Here's the drawing with two shaded views (mm, measured from the low corner). I have some questions. A direction names the side the tool comes from. Coordinates: 2 decimals unless noted, no trailing zeros. Order: outer loops, then holes, each group sorted by start corner. A loop starts at its lowest first (then second) coordinate and runs counter-clockwise, first axis right, second up. Notation, with made-up numbers: (9.25, 84) - (56.25, 84) arc R29 cw to (56.25, 117) - close; hole circle Ø4 at (13, 47.5). An arc over 180 degrees is marked (long way). Answer as CSV lines item,"result". Start each with the question number.
1. I want a section at D-D, the plane z = 9. List the corners of the cut face in (x, y) for me, and give its area (3 significant figures).
2. I want a section at B-B, the plane y = 20. List the corners of the cut face in (x, z) for me, and give its area (3 significant figures).
3. Thinking about a two-plate mould opening in X: for the marked faces 1, 2, 3 and 4, which applies, released by +X, released by -X, zero draft, split by the parting line, or undercut?
4. For the marked faces 5 and 6, which set-ups out of +Z, -Z, +X, -X, +Y, -Y let a thin tool reach every point of the face, with its end or its side?
5. I want a section at A-A, the plane x = 40.5. List the corners of the cut face in (y, z) for me.
6. I want a section at C-C, the plane y = 24.5. List the corners of the cut face in (x, z) for me.
7. I need wall thicknesses on probe 1 along Y at (x, z) = (20, 6.75); probe 2 along X at (y, z) = (22.5, 6); probe 3 along X at (y, z) = (38.5, 9). Which ranges of each line are inside material? Lowest first, please.
8. For pin 1 (0.9 mm diameter, centred on x = 41.5, z = 5.5, fed in from -Y); pin 2 (4 mm diameter, centred on x = 43.5, z = 5.5, fed in from +Y); pin 3 (5 mm diameter, centred on y = 5, z = 2.5, fed in from +X), each with a flat end and sliding along its axis, tell me the tip position at first contact or that it passes through.
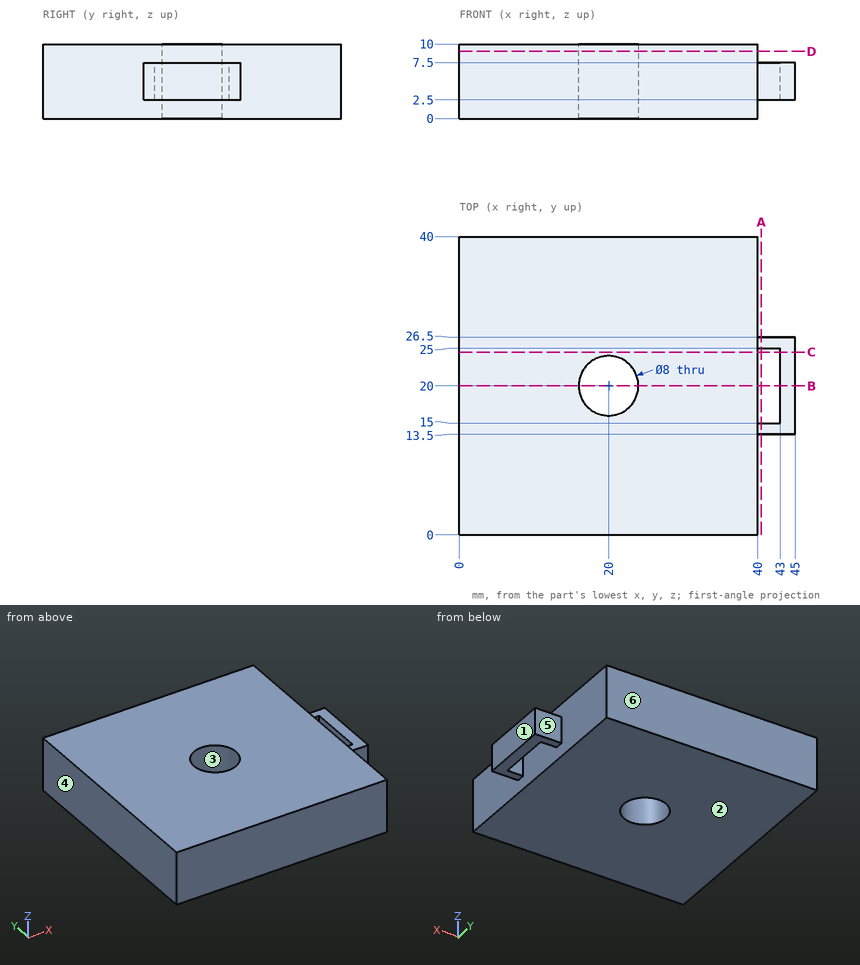
Solved:
1,outline,"(0, 0) - (40, 0) - (40, 40) - (0, 40) - close; hole circle Ø8 at (20, 20)"
1,area,"1,550 mm2"
2,outline,"(0, 0) - (16, 0) - (16, 10) - (0, 10) - close; (24, 0) - (40, 0) - (40, 10) - (24, 10) - close; (43, 2.5) - (45, 2.5) - (45, 7.5) - (43, 7.5) - close"
2,area,"330 mm2"
3,face 1,"released by +X"
3,face 2,"zero draft"
3,face 3,"undercut"
3,face 4,"released by -X"
4,face 5,"+Z, -Z, +X, +Y"
4,face 6,"+Z, -Z, +X, -X, +Y"
5,outline,"(13.5, 2.5) - (15, 2.5) - (15, 7.5) - (13.5, 7.5) - close; (25, 2.5) - (26.5, 2.5) - (26.5, 7.5) - (25, 7.5) - close"
6,outline,"(0, 0) - (40, 0) - (40, 10) - (0, 10) - close; (43, 2.5) - (45, 2.5) - (45, 7.5) - (43, 7.5) - close"
7,probe 1,"y = 0 to 16, 24 to 40"
7,probe 2,"x = 0 to 16.88, 23.12 to 40, 43 to 45"
7,probe 3,"x = 0 to 40"
8,pin 1,"stops at y = 13.5"
8,pin 2,"stops at y = 26.5"
8,pin 3,"stops at x = 40"
